Source: CAD feature listing. Evaluate the final solid. Frame: model axes, mm. Round coordinates to 2 decimals unless told otherwise and drop trailing zeros. Loops run counter-clockwise (first coordinate to the right, second up) from the corner with the lowest first, then second, coordinate; pieces in that order, holes last. Notation, with made-up numbers: M -39,55 L -26,55 A24 ccw -26,82 Z; hole C -35.5,54 d4. An arc over 180 degrees is marked long. Answer as a JSON object with one key per item and string values.
from build123d import *

# Parameters (mm, degrees)
BOSS_EXTRUDE1_DEPTH = 2.2
CUT_EXTRUDE1_REACH  = 178.497
SKETCH4_R           = 1.5
CUT_EXTRUDE2_REACH  = 178.497
SKETCH5_R           = 1.5


with BuildPart() as part:
    # Sketch2 → Boss-Extrude1 (new body)
    with BuildSketch(Plane.XY):
        with BuildLine():
            Line((-121.5, 0), (-36.5, 0))
            ThreePointArc((-36.5, 0), (1.5, -40), (39.5, 0))
            Line((39.5, 0), (120.5, 0))
            Line((120.5, 0), (120.5, -55))
            ThreePointArc((120.5, -55), (0.955998142, -127.970310059), (-121.5, -60))
            Line((-121.5, -60), (-121.5, 0))
        make_face()
    extrude(amount=BOSS_EXTRUDE1_DEPTH)

    # Sketch4 → Cut-Extrude1 (cut, up to next)
    with BuildSketch(Plane.XY.offset(2.2), mode=Mode.PRIVATE) as cut_extrude1_sk1:
        with Locations((109.5, -9)):
            Circle(SKETCH4_R)
    cut_extrude1_tool1 = extrude(cut_extrude1_sk1.sketch, amount=-CUT_EXTRUDE1_REACH, mode=Mode.PRIVATE) & part.part
    # Sketch4 → Cut-Extrude1 (cut, up to next)
    with BuildSketch(Plane.XY.offset(2.2), mode=Mode.PRIVATE) as cut_extrude1_sk2:
        with Locations((49.5, -9)):
            Circle(SKETCH4_R)
    cut_extrude1_tool2 = extrude(cut_extrude1_sk2.sketch, amount=-CUT_EXTRUDE1_REACH, mode=Mode.PRIVATE) & part.part
    # Sketch4 → Cut-Extrude1 (cut, up to next)
    with BuildSketch(Plane.XY.offset(2.2), mode=Mode.PRIVATE) as cut_extrude1_sk3:
        with Locations((-45.5, -9)):
            Circle(SKETCH4_R)
    cut_extrude1_tool3 = extrude(cut_extrude1_sk3.sketch, amount=-CUT_EXTRUDE1_REACH, mode=Mode.PRIVATE) & part.part
    # Sketch4 → Cut-Extrude1 (cut, up to next)
    with BuildSketch(Plane.XY.offset(2.2), mode=Mode.PRIVATE) as cut_extrude1_sk4:
        with Locations((-112.5, -9)):
            Circle(SKETCH4_R)
    cut_extrude1_tool4 = extrude(cut_extrude1_sk4.sketch, amount=-CUT_EXTRUDE1_REACH, mode=Mode.PRIVATE) & part.part
    add(cut_extrude1_tool1.solids().sort_by_distance((109.5, -9, 2.2))[0], mode=Mode.SUBTRACT)
    add(cut_extrude1_tool2.solids().sort_by_distance((49.5, -9, 2.2))[0], mode=Mode.SUBTRACT)
    add(cut_extrude1_tool3.solids().sort_by_distance((-45.5, -9, 2.2))[0], mode=Mode.SUBTRACT)
    add(cut_extrude1_tool4.solids().sort_by_distance((-112.5, -9, 2.2))[0], mode=Mode.SUBTRACT)

    # Sketch5 → Cut-Extrude2 (cut, up to next)
    with BuildSketch(Plane.XY.offset(2.2), mode=Mode.PRIVATE) as cut_extrude2_sk1:
        with Locations((114.5, -34)):
            Circle(SKETCH5_R)
    cut_extrude2_tool1 = extrude(cut_extrude2_sk1.sketch, amount=-CUT_EXTRUDE2_REACH, mode=Mode.PRIVATE) & part.part
    # Sketch5 → Cut-Extrude2 (cut, up to next)
    with BuildSketch(Plane.XY.offset(2.2), mode=Mode.PRIVATE) as cut_extrude2_sk2:
        with Locations((114.5, -54)):
            Circle(SKETCH5_R)
    cut_extrude2_tool2 = extrude(cut_extrude2_sk2.sketch, amount=-CUT_EXTRUDE2_REACH, mode=Mode.PRIVATE) & part.part
    # Sketch5 → Cut-Extrude2 (cut, up to next)
    with BuildSketch(Plane.XY.offset(2.2), mode=Mode.PRIVATE) as cut_extrude2_sk3:
        with Locations((36.5, -34)):
            Circle(SKETCH5_R)
    cut_extrude2_tool3 = extrude(cut_extrude2_sk3.sketch, amount=-CUT_EXTRUDE2_REACH, mode=Mode.PRIVATE) & part.part
    # Sketch5 → Cut-Extrude2 (cut, up to next)
    with BuildSketch(Plane.XY.offset(2.2), mode=Mode.PRIVATE) as cut_extrude2_sk4:
        with Locations((36.5, -54)):
            Circle(SKETCH5_R)
    cut_extrude2_tool4 = extrude(cut_extrude2_sk4.sketch, amount=-CUT_EXTRUDE2_REACH, mode=Mode.PRIVATE) & part.part
    add(cut_extrude2_tool1.solids().sort_by_distance((114.5, -34, 2.2))[0], mode=Mode.SUBTRACT)
    add(cut_extrude2_tool2.solids().sort_by_distance((114.5, -54, 2.2))[0], mode=Mode.SUBTRACT)
    add(cut_extrude2_tool3.solids().sort_by_distance((36.5, -34, 2.2))[0], mode=Mode.SUBTRACT)
    add(cut_extrude2_tool4.solids().sort_by_distance((36.5, -54, 2.2))[0], mode=Mode.SUBTRACT)


solid = part.part
Item 1: Section A-A on z = 1.5. Give the number of separate pieces and of enclosed holes in the cut face, then the cut area to 3 significant figures.
Answer sheet:
{"separate pieces": "1", "enclosed holes": "8", "area": "23,500 mm²"}
Item 2: Contact query for a flat-ended pin moving along its axis: pin 1 Ø1 at (x, z) = (-69.5, 1) entering from -Y. Output: stop coordinate, or through.
Answer sheet:
{"pin 1": "stops at y = -110.76"}
Item 3: Section C-C on y = -91. Return the cut outline in (x, z), then the cut area to 3 significant figures.
Answer sheet:
{"outline": "M -96.41,0 L 92.57,0 L 92.57,2.2 L -96.41,2.2 Z", "area": "416 mm²"}
Item 4: Line query: probe 1 along Y at (x, z) = (36.5, 0.75); probe 2 along X at (y, z) = (-34.5, 1.35); probe 3 along Y at (x, z) = (114.5, 1.65). Output: solid intervals per line, ascending. Write a range as from..to.
Answer sheet:
{"probe 1": "y = -122.59..-55.5, -52.5..-35.5, -32.5..-16.88", "probe 2": "x = -121.5..-18.21, 21.21..35.09, 37.91..113.09, 115.91..120.5", "probe 3": "y = -65.07..-55.5, -52.5..-35.5, -32.5..0"}
Item 5: Section B-B on x = 13.5. Return the cut outline in (y, z), then the cut area to 3 significant figures.
Answer sheet:
{"outline": "M -127.14,0 L -38.06,0 L -38.06,2.2 L -127.14,2.2 Z", "area": "196 mm²"}
Item 6: Pull-direction query (X, two-part tool) for faces 1 (the cylindrical face through (3.01, -127.913, 1.085)), 2 (the flat face through (1, -63, 0)), 3 (the cylindrical face through (0.64, -39.99, 1.08)); classes: pulls with the +X half, pulls with the -X half, needs draft (parallel to the pull), parting line crosses it, or undercut.
Answer sheet:
{"face 1": "parting line crosses it", "face 2": "needs draft", "face 3": "undercut"}
